Build history of the part. All positions in model axes, mm. A direction names the side the tool comes from. Coordinates: 2 decimals unless noted, no trailing zeros. Order: outer loops, then holes, each group sorted by start corner. A loop starts at its lowest first (then second) coordinate and runs counter-clockwise, first axis right, second up. Notation, with made-up numbers: M 46,76 L 62,76 A18 ccw 62,94 Z; hole C -34,26 d1. An arc over 180 degrees is marked long. Write item = value, one per line. Start each with the question number.
Q1. Pin check, flat tip, straight feed: P1, Ø4, axis at x = -3, y = -4, coming from the -Z side. Stop position of the tip, or through.
Q2. Band-saw the part on A-A on y = -4. Write the cut outline in (x, z), plus the area to 3 significant figures.
Q3. Band-saw the part on B-B on x = -4. Write the cut outline in (y, z).
Q4. Pull direction Y, two halves, no side cores. Call faces 3 (the face through (9.4, -6.93, 2.89)), 4 (the face through (-9.29, -6.82, 2.89)), 5 (the face through (-9.4, 6.93, 2.89)): released by +Y, released by -Y, zero draft, split by the parting line, or undercut.
Q5. 3-axis set-ups, long thin cutter, end or side, ignore diameter. For faces 1 (the face through (9.43, 6.9, 2.89)), 2 (the face through (9.32, -6.79, 2.89)): which of +Z, -Z, +X, -X, +Y, -Y reach the whole face in a straight line?
Q6. Band-saw the part on D-D on x = 8.75. Write the cut outline in (y, z), plus the area to 3 significant figures.
Q7. Drill centre lines: probe 1 along X at (y, z) = (6.5, 3.5); probe 2 along Y at (x, z) = (9, 20); probe 3 along X at (y, z) = (6.75, 26.5). Where is each one in solid material? Low to high.
Q8. Band-saw the part on C-C on z = 24.5. Write the cut outline in (x, y), plus the area to 3 significant figures.
```python
from build123d import *

# Parameters (mm, degrees)
F1_DEPTH = 30
F2_W     = 15.78
F2_H     = 0.11
F3_DEPTH = 5
F4_W     = 15.78
F4_H     = 0.11
F5_DEPTH = 4.9
F6_DEPTH = 25


with BuildPart() as f1:
    # F0 (on Top) → F1 (new body)
    with BuildSketch(Plane.XY):
        with BuildLine():
            Line((-8, -7.5), (8, -7.5))
            ThreePointArc((8, -7.5), (9.4142135624, -6.9142135624), (10, -5.5))
            Line((10, -5.5), (10, 5.5))
            ThreePointArc((10, 5.5), (9.4142135624, 6.9142135624), (8, 7.5))
            Line((8, 7.5), (-8, 7.5))
            ThreePointArc((-8, 7.5), (-9.4142135624, 6.9142135624), (-10, 5.5))
            Line((-10, 5.5), (-10, -5.5))
            ThreePointArc((-10, -5.5), (-9.4142135624, -6.9142135624), (-8, -7.5))
        make_face()
        with BuildLine():
            Line((-7.89, 7.39), (7.89, 7.39))
            ThreePointArc((7.89, 7.39), (9.3042135624, 6.8042135624), (9.89, 5.39))
            Line((9.89, 5.39), (9.89, -5.39))
            ThreePointArc((9.89, -5.39), (9.3042135624, -6.8042135624), (7.89, -7.39))
            Line((7.89, -7.39), (-7.89, -7.39))
            ThreePointArc((-7.89, -7.39), (-9.3042135624, -6.8042135624), (-9.89, -5.39))
            Line((-9.89, -5.39), (-9.89, 5.39))
            ThreePointArc((-9.89, 5.39), (-9.3042135624, 6.8042135624), (-7.89, 7.39))
        make_face(mode=Mode.SUBTRACT)
    extrude(amount=F1_DEPTH)

    # F2 (on face) → F3 (join)
    with BuildSketch(Plane.XZ.offset(-7.39)):
        with Locations((0, 29.945)):
            Rectangle(F2_W, F2_H)
    extrude(amount=F3_DEPTH)

    # F4 (on face) → F5 (join)
    with BuildSketch(Plane(origin=(0, -7.39, 0), x_dir=(-1, 0, 0), z_dir=(0, 1, 0))):
        with Locations((0, 29.945)):
            Rectangle(F4_W, F4_H)
    extrude(amount=F5_DEPTH)

    # F6 (add): a face of the model
    f6_faces = [f1.faces().sort_by_distance(p)[0] for p in [
        (0, -7.475, 0),
    ]]
    extrude(f6_faces, amount=F6_DEPTH)


solid = f1.part
```
Recorded:
q1.P1 = 29.89
q2.outline = M -10,-25 L -9.89,-25 L -9.89,30 L -10,30 Z; M -7.89,29.89 L 7.89,29.89 L 7.89,30 L -7.89,30 Z; M 9.89,-25 L 10,-25 L 10,30 L 9.89,30 Z
q2.area = 13.8 mm2
q3.outline = M -7.5,-25 L -7.39,-25 L -7.39,29.89 L -2.49,29.89 L -2.49,30 L -7.5,30 Z; M 2.39,29.89 L 7.39,29.89 L 7.39,-25 L 7.5,-25 L 7.5,30 L 2.39,30 Z
q4.face_3 = released by -Y
q4.face_4 = undercut
q4.face_5 = released by +Y
q5.face_1 = +Z, -Z, +X, +Y
q5.face_2 = +Z, -Z
q6.outline = M -7.35,-25 L -7.2,-25 L -7.2,30 L -7.35,30 Z; M 7.2,-25 L 7.35,-25 L 7.35,30 L 7.2,30 Z
q6.area = 17.4 mm2
q7.probe_1 = -9.73 to -9.55, 9.55 to 9.73
q7.probe_2 = -7.23 to -7.05, 7.05 to 7.23
q7.probe_3 = -9.56 to -9.36, 9.36 to 9.56
q8.outline = M -10,-5.5 A2 ccw -8,-7.5 L 8,-7.5 A2 ccw 10,-5.5 L 10,5.5 A2 ccw 8,7.5 L -8,7.5 A2 ccw -10,5.5 Z; hole M -9.89,-5.39 A2 ccw -7.89,-7.39 L 7.89,-7.39 A2 ccw 9.89,-5.39 L 9.89,5.39 A2 ccw 7.89,7.39 L -7.89,7.39 A2 ccw -9.89,5.39 Z
q8.area = 7.65 mm2
